Can you work these out from the model? Positions are in its coordinate system, mm. Face numbers are marked on the shaded views. Round coordinates to 2 decimals unless told otherwise and drop trailing zeros. Loops run counter-clockwise (first coordinate to the right, second up) from the corner with the lowest first, then second, coordinate; pieces in that order, holes last.
(1) If I drill on line 1 along Z through (x, y) = (0, 3.15); line 2 along Z through (x, y) = (0.05, -3.75), over which ranges is the centre line in solid material (lowest first)?
(2) Thinking about a two-plate mould opening in X: for the marked faces 1, 2 and 3, which applies, released by +X, released by -X, zero draft, split by the parting line, or undercut?
(3) I want a section at A-A on x = 0. Write out the boundary of the cut face in (y, z), plus the area to 3 significant figures.
(4) Will these pins go through, and if not, where does the flat tip stop? pin 1 Ø3 at (y, z) = (-3.5, 2) entering from +X; pin 2 Ø3 at (y, z) = (-4.5, 0) entering from +X; pin 3 Ø3 at (y, z) = (-4.5, -1) entering from -X.
(5) I want a section at D-D on z = 1.3. Write out the boundary of the cut face in (x, y), plus the area to 3 significant figures.
(6) I want a section at B-B on z = 0. Write out the boundary of the cut face in (x, y).
(7) I want a section at C-C on y = 2. Write out the boundary of the cut face in (x, z).
Autodesk Inventor part; units mm, degrees
ref_plane "YZ Plane" through (0, 0, 0) normal (1, 0, 0) x (0, 1, 0)
ref_plane "XZ Plane" through (0, 0, 0) normal (0, 1, 0) x (-1, 0, 0)
ref_plane "XY Plane" through (0, 0, 0) normal (0, 0, 1) x (1, 0, 0)
sketch "Sketch1" plane through (0, 0, 0) normal (0, 1, 0) x (-1, 0, 0)
  circle A0 centre (0, 0) radius 3
  circle A1 centre (0, 0) radius 2.5
  dimension "d0" = 6
  dimension "d1" = 5
extrude "Extrusion1" add sketch "Sketch1" along normal blind 6
sketch "Sketch2" plane through (0, 0, 0) normal (0, -1, 0) x (1, 0, 0)
  circle A0 centre (0, 0) radius 1
  circle A1 centre (0, 0) radius 3
  dimension "d6" = 2
extrude "Extrusion2" add sketch "Sketch2" along normal blind 1
sketch "Sketch3" plane through (0, -1, 0) normal (0, -1, 0) x (1, 0, 0)
  circle A0 centre (0, 0) radius 1.5
  circle A1 centre (0, 0) radius 1
  dimension "d9" = 3
extrude "Extrusion3" add sketch "Sketch3" along normal blind 5
thread "Thread2"
properties part number "NozzleAttachment"
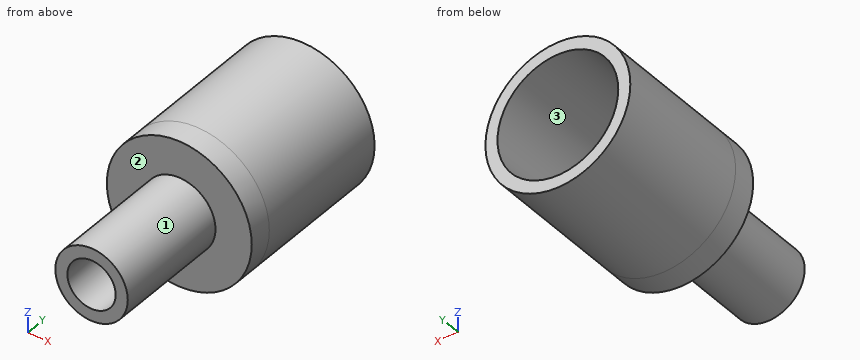
Filled sheet:
1. line 1: z = -3 to -2.5, 2.5 to 3
1. line 2: z = -1.5 to -1, 1 to 1.5
2. face 1: split by the parting line
2. face 2: zero draft
2. face 3: undercut
3. outline: (-6, -1.5) - (-1, -1.5) - (-1, -3) - (6, -3) - (6, -2.5) - (0, -2.5) - (0, -1) - (-6, -1) - close; (-6, 1) - (0, 1) - (0, 2.5) - (6, 2.5) - (6, 3) - (-1, 3) - (-1, 1.5) - (-6, 1.5) - close
3. area: 15.0 mm2
4. pin 1: stops at x = 1.41
4. pin 2: stops at x = 1.5
4. pin 3: stops at x = -1.5
5. outline: (-2.7, -1) - (-0.75, -1) - (-0.75, -6) - (0.75, -6) - (0.75, -1) - (2.7, -1) - (2.7, 6) - (2.14, 6) - (2.14, 0) - (-2.14, 0) - (-2.14, 6) - (-2.7, 6) - close
5. area: 19.7 mm2
6. outline: (-3, -1) - (-1.5, -1) - (-1.5, -6) - (-1, -6) - (-1, 0) - (-2.5, 0) - (-2.5, 6) - (-3, 6) - close; (1, -6) - (1.5, -6) - (1.5, -1) - (3, -1) - (3, 6) - (2.5, 6) - (2.5, 0) - (1, 0) - close
7. outline: circle Ø6 at (0, 0); hole circle Ø5 at (0, 0)
